```python
from build123d import *

# Parameters (mm, degrees)
F0_W     = 25.4
F0_H     = 70.3412795041
F1_DEPTH = 50.8


with BuildPart() as f1:
    # F0 (on Front) → F1 (new body, symmetric)
    with BuildSketch(Plane.XZ):
        with Locations((-50.3423148662, -42.8482267274)):
            Rectangle(F0_W, F0_H)
        Polygon((76.6576851338, 58.313548793), (-24.9423148662, 58.313548793), (-63.0423148662, -7.6775869753), (-37.6423148662, -7.6775869753), (89.3576851338, -7.6775869753), (114.7576851338, -7.6775869753), align=None)
        with Locations((102.0576851338, -42.8482267274)):
            Rectangle(F0_W, F0_H)
    extrude(amount=F1_DEPTH, both=True)


solid = f1.part
```
Design review of the part built by this model. Coordinates are the model's own, in mm. A direction names the side the tool comes from. Give positions to 0.01 mm unless a question says otherwise; leave off trailing zeros. Loops run counter-clockwise (first coordinate to the right, second up) from the corner with the lowest first, then second, coordinate; pieces in that order, holes last. Notation, with made-up numbers: (30.5, 86.25) -> (62.5, 86.25) arc R23 cw to (62.5, 106.25) -> close; hole circle Ø8 at (12.5, 83.25). An arc over 180 degrees is marked (long way). One line per item, written item: value.
Q1. For pin 1 Ø1 at (x, y) = (16.5, 26) entering from -Z, flat-tipped, find the tip position at first contact; note if it passes through.
Numbers:
pin 1: stops at z = -7.68
Q2. We need section C-C on x = 27.5. Give the boundary of the cut face in (y, z).
Numbers:
outline: (-50.8, -7.68) -> (50.8, -7.68) -> (50.8, 58.31) -> (-50.8, 58.31) -> close
Q3. For L1, parallel to X at y = -22, z = -31; L2, parallel to Z at x = 59, y = 36; L3, parallel to X at y = -19.5, z = 48, list the stretches that pass through material, from the lowest coordinate up.
Numbers:
L1: x = -63.04 to -37.64, 89.36 to 114.76
L2: z = -7.68 to 58.31
L3: x = -30.9 to 82.61
Q4. We need section A-A on z = -14. Give the boundary of the cut face in (x, y), and give its area (3 significant figures).
Numbers:
outline: (-63.04, -50.8) -> (-37.64, -50.8) -> (-37.64, 50.8) -> (-63.04, 50.8) -> close; (89.36, -50.8) -> (114.76, -50.8) -> (114.76, 50.8) -> (89.36, 50.8) -> close
area: 5,160 mm^2
Q5. Machinability: for faces 4 (the flat face through (25, -50.8, 6)), 5 (the flat face through (25, -1, -7.678)), which of the approach directions +Z, -Z, +X, -X, +Y, -Y give a long, thin tool a straight path to every point of the face, cutting with its end or side? Answer none if there is none.
Numbers:
face 4: +Z, -Z, +X, -X, -Y
face 5: -Z, +Y, -Y
Q6. Draft analysis for pull direction X (two halves, no side actions). For faces 1 (the flat face through (25, 50.8, 6)), 2 (the flat face through (89.358, -1, -43)), 3 (the flat face through (-63.042, -1, -43)), state which applies: pulls with the +X half, pulls with the -X half, needs draft (parallel to the pull), parting line crosses it, or undercut.
Numbers:
face 1: needs draft
face 2: undercut
face 3: pulls with the -X half
Q7. We need section B-B on y = -10. Give the boundary of the cut face in (x, z), and give its area (3 significant figures).
Numbers:
outline: (-63.04, -78.02) -> (-37.64, -78.02) -> (-37.64, -7.68) -> (89.36, -7.68) -> (89.36, -78.02) -> (114.76, -78.02) -> (114.76, -7.68) -> (76.66, 58.31) -> (-24.94, 58.31) -> (-63.04, -7.68) -> close
area: 12,800 mm^2
Q8. We need section D-D on z = 10.5. Give the boundary of the cut face in (x, y).
Numbers:
outline: (-52.55, -50.8) -> (104.26, -50.8) -> (104.26, 50.8) -> (-52.55, 50.8) -> close
